The listing builds one solid part. Answer for the finished solid, in the listing's coordinates (mm). A direction names the side the tool comes from. Give positions to 0.01 mm unless a question says otherwise; leave off trailing zeros. Order: outer loops, then holes, each group sorted by start corner. A loop starts at its lowest first (then second) coordinate and runs counter-clockwise, first axis right, second up. Notation, with made-up numbers: (11, -22.75) -> (36, -22.75) arc R10 cw to (36, -9.75) -> close; hole circle Ø4 at (73.25, 31.5). An arc over 180 degrees is marked (long way). One line per question, with ' | ' between items. Start each with the question number.
```python
from build123d import *


with BuildPart() as part:
    # Sketch1 → Revolve1 (revolve)
    with BuildSketch(Plane(origin=(0, 0, 0), x_dir=(0, 0, -1), z_dir=(1, 0, 0))):
        with BuildLine():
            Line((0.635, 7.62), (1.1938, 7.62))
            Line((1.1938, 7.62), (1.1938, 5.08))
            Line((1.1938, 5.08), (1.905, 5.08))
            Line((1.905, 5.08), (1.905, 4.318))
            Line((1.905, 4.318), (1.0922, 4.318))
            Line((1.0922, 4.318), (1.0922, 0))
            Line((1.0922, 0), (0, 0))
            Line((0, 0), (0, 9.906))
            ThreePointArc((0, 9.906), (0.449012806, 9.720012806), (0.635, 9.271))
            Line((0.635, 9.271), (0.635, 7.62))
        make_face()
    revolve(axis=Axis((0, 0, 0), (0, 1, 0)))


solid = part.part
```
(1) For faces 1 (the face through (1.86, 4.69, 0.41)), 2 (the face through (1, 7.62, 0)), 3 (the face through (-0.33, 2.13, -1.04)), determine the directions among +Z, -Z, +X, -X, +Y, -Y from which every point of the face is accessible in a straight line to the end or side of a thin tool.
(2) The part is cut by section B-B on x = 0. Determine the outline of the cut face in (y, z) (3 decimals), plus the area to 3 significant figures.
(3) Consider line 1 (Z direction, x = -0.05, y = 1.5); line 2 (Y direction, x = 1.65, z = 0.55); line 3 (X direction, y = 6.25, z = 0.05). Determine where each line is inside the solid, lowest interval first.
(4) The part is cut by section A-A on z = -0.25. Determine the outline of the cut face in (x, y), plus the area to 3 significant figures.
(5) The part is cut by section D-D on x = 1.65. Determine the outline of the cut face in (y, z).
(6) Given P1, Ø1.5, axis at y = 4.5, z = -0.5, coming from the +X side (3 decimals); P2, Ø1, axis at y = 5.5, z = 1, coming from the +X side; P3, Ø1, axis at y = 6, z = 0, coming from the -X side; P4, Ø2, axis at x = -1.5, y = 2.5, coming from the +Z side, each flat-ended and moving along its own axis, determine where each tip first touches the part or whether it passes through.
(7) The part is cut by section C-C on y = 7.75. Determine the outline of the cut face in (x, z) (3 decimals), plus the area to 3 significant figures.
Result sheet:
1) face 1: +Y, -Y | face 2: +Y | face 3: -Y
2) outline: (0, -1.092) -> (4.318, -1.092) -> (4.318, -1.905) -> (5.08, -1.905) -> (5.08, -1.194) -> (7.62, -1.194) -> (7.62, -0.635) -> (9.271, -0.635) arc R0.635 ccw to (9.271, 0.635) -> (7.62, 0.635) -> (7.62, 1.194) -> (5.08, 1.194) -> (5.08, 1.905) -> (4.318, 1.905) -> (4.318, 1.092) -> (0, 1.092) -> close | area: 21.1 mm^2
3) line 1: z = -1.09 to 1.09 | line 2: y = 4.32 to 5.08 | line 3: x = -1.19 to 1.19
4) outline: (-1.89, 4.32) -> (-1.06, 4.32) -> (-1.06, 0) -> (1.06, 0) -> (1.06, 4.32) -> (1.89, 4.32) -> (1.89, 5.08) -> (1.17, 5.08) -> (1.17, 7.62) -> (0.58, 7.62) -> (0.58, 9.27) arc R0.58 ccw to (-0.58, 9.27) -> (-0.58, 7.62) -> (-1.17, 7.62) -> (-1.17, 5.08) -> (-1.89, 5.08) -> close | area: 20.5 mm^2
5) outline: (4.32, -0.95) -> (5.08, -0.95) -> (5.08, 0.95) -> (4.32, 0.95) -> close
6) P1: stops at x = 1.905 | P2: stops at x = 1.76 | P3: stops at x = -1.19 | P4: stops at z = 0.97
7) outline: circle Ø1.27 at (0, 0) | area: 1.27 mm^2
